from build123d import *

# Parameters (mm, degrees)
SKETCH1_W               = 60
SKETCH1_H               = 150
BOSS_EXTRUDE1_DEPTH     = 150
CUT_EXTRUDE1_DEPTH      = 100
CUT_EXTRUDE1_DEPTH_BACK = 100
SKETCH2_R               = 10
CUT_EXTRUDE2_DEPTH      = 100
CUT_EXTRUDE2_DEPTH_BACK = 100
SKETCH3_W               = 100
SKETCH3_H               = 80
SKETCH5_W               = 25
SKETCH5_H               = 25
BOSS_EXTRUDE3_DEPTH     = 25
SKETCH6_R               = 7.5
BOSS_EXTRUDE4_DEPTH     = 10


with BuildPart() as part:
    # Sketch1 → Boss-Extrude1 (new body)
    with BuildSketch(Plane(origin=(0, 0, 0), x_dir=(1, 0, 0), z_dir=(0, 1, 0))):
        Rectangle(SKETCH1_W, SKETCH1_H)
    extrude(amount=BOSS_EXTRUDE1_DEPTH)

    # Sketch2 → Cut-Extrude1 (cut, two sides: drawn at the far end of the back side and taken through both)
    with BuildSketch(Plane.XY.offset(-CUT_EXTRUDE1_DEPTH_BACK)):
        with Locations(Location((0, 15, 0), (0, 0, 180))):
            Circle(SKETCH2_R)
    extrude(amount=CUT_EXTRUDE1_DEPTH + CUT_EXTRUDE1_DEPTH_BACK, mode=Mode.SUBTRACT)

    # Sketch3 → Cut-Extrude2 (cut, two sides: drawn at the far end of the back side and taken through both)
    with BuildSketch(Plane(origin=(0, 0, 0), x_dir=(0, 0, -1), z_dir=(1, 0, 0)).offset(-CUT_EXTRUDE2_DEPTH_BACK)):
        Rectangle(SKETCH3_W, SKETCH3_H)
    extrude(amount=CUT_EXTRUDE2_DEPTH + CUT_EXTRUDE2_DEPTH_BACK, mode=Mode.SUBTRACT)

    # Sketch5 → Boss-Extrude3 (add)
    with BuildSketch(Plane(origin=(0, 150, 0), x_dir=(1, 0, 0), z_dir=(0, 1, 0))):
        with Locations((0, 50)):
            Rectangle(SKETCH5_W, SKETCH5_H)
    extrude(amount=BOSS_EXTRUDE3_DEPTH)

    # Sketch6 → Boss-Extrude4 (add)
    with BuildSketch(Plane(origin=(12.5, 0, 0), x_dir=(0, 0, -1), z_dir=(1, 0, 0))):
        with Locations(Location((50, 162.5, 0), (0, 0, 180))):
            Circle(SKETCH6_R)
    extrude(amount=BOSS_EXTRUDE4_DEPTH)


solid = part.part
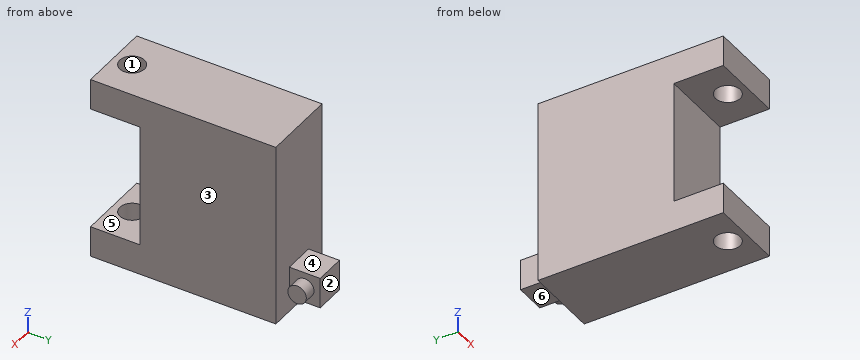
The listing builds one solid part. Answer for the finished solid, in the listing's coordinates (mm). Face numbers are marked on the shaded views. A direction names the side the tool comes from. Round coordinates to 2 decimals unless told otherwise and drop trailing zeros. Order: outer loops, then holes, each group sorted by start corner. A loop starts at its lowest first (then second) coordinate and runs counter-clockwise, first axis right, second up. Notation, with made-up numbers: (31.25, -25) -> (54.25, -25) arc R19 cw to (54.25, -5) -> close; hole circle Ø4 at (56.25, 39). An arc over 180 degrees is marked (long way). One line per item, written item: value.
Item 1: Find section A-A, the plane y = 15. Give the vertices of the cut face in (x, z), then the cut area to 3 significant figures.
Taken from the geometry:
outline: (-30, -75) -> (-10, -75) -> (-10, -50) -> (-30, -50) -> close; (-30, 50) -> (-10, 50) -> (-10, 75) -> (-30, 75) -> close; (10, -75) -> (30, -75) -> (30, -50) -> (10, -50) -> close; (10, 50) -> (30, 50) -> (30, 75) -> (10, 75) -> close
area: 2,000 mm2
Item 2: Straight lines are drawn through the part: L1, parallel to Z at x = 11.5, y = 13; L2, parallel to Y at x = 0, z = 58; L3, parallel to Y at x = 0, z = -57. For each, find the intervals that lie inside material, in ascending order.
Taken from the geometry:
L1: z = -75 to -50, 50 to 75
L2: y = 0 to 5, 25 to 150
L3: y = 0 to 5, 25 to 175
Item 3: Find section B-B, the plane x = 0. Give the vertices of the cut face in (y, z).
Taken from the geometry:
outline: (0, -75) -> (5, -75) -> (5, -50) -> (0, -50) -> close; (0, 50) -> (5, 50) -> (5, 75) -> (0, 75) -> close; (25, -75) -> (150, -75) -> (150, -62.5) -> (175, -62.5) -> (175, -37.5) -> (150, -37.5) -> (150, 75) -> (25, 75) -> (25, 50) -> (40, 50) -> (40, -50) -> (25, -50) -> close
Item 4: Find section C-C, the plane z = -59.5. Give the vertices of the cut face in (x, y).
Taken from the geometry:
outline: (-30, 0) -> (30, 0) -> (30, 150) -> (12.5, 150) -> (12.5, 175) -> (-12.5, 175) -> (-12.5, 150) -> (-30, 150) -> close; hole circle Ø20 at (0, 15)
Item 5: Find section D-D, the plane x = -18. Give the vertices of the cut face in (y, z), then the cut area to 3 significant figures.
Taken from the geometry:
outline: (0, -75) -> (150, -75) -> (150, 75) -> (0, 75) -> (0, 50) -> (40, 50) -> (40, -50) -> (0, -50) -> close
area: 18,500 mm2
Item 6: For a pull along Y with two mould halves and no side action, classify the marked faces 1, 2 and 3 as released by +Y, released by -Y, zero draft, split by the parting line, or undercut.
Taken from the geometry:
face 1: undercut
face 2: released by +Y
face 3: zero draft
Item 7: Given P1, Ø3, axis at x = 21.5, z = -48, coming from the +Y side; P2, Ø20, axis at y = 156.5, z = -54, coming from the -X side; P3, Ø12, axis at y = 160.5, z = -53, coming from the +X side; P4, Ø12.5, axis at x = -2.5, y = 165.5, coming from the +Z side, each flat-ended and moving along its own axis, determine where each tip first touches the part or whether it passes through.
Taken from the geometry:
P1: stops at y = 169.98
P2: stops at x = -30
P3: stops at x = 22.5
P4: stops at z = -37.5
Item 8: For the marked faces 4, 5 and 6, determine the directions among +Z, -Z, +X, -X, +Y, -Y from which every point of the face is accessible in a straight line to the end or side of a thin tool.
Taken from the geometry:
face 4: +Z, +X, -X, +Y
face 5: +X, -X, -Y
face 6: -Z, +X, -X, +Y
